Build history of the part. All positions in model axes, mm. Face numbers are marked on the shaded views. A direction names the side the tool comes from. Round coordinates to 2 decimals unless told otherwise and drop trailing zeros. Order: outer loops, then holes, each group sorted by start corner. A loop starts at its lowest first (then second) coordinate and runs counter-clockwise, first axis right, second up. Notation, with made-up numbers: (63, 81.25) -> (91, 81.25) arc R18 cw to (91, 98.25) -> close; hole circle Ø5 at (32.25, 85.5). An arc over 180 degrees is marked (long way). Answer as a JSON object with one key per item and string values.
from build123d import *

# Parameters (mm, degrees)
ESTRUSIONE_ESTRUSIONE1_DEPTH = 100
ESTRUSIONE_ESTRUSIONE2_DEPTH = 3


with BuildPart() as part:
    # Schizzo1 → Estrusione-Estrusione1 (new body)
    with BuildSketch(Plane(origin=(0, 0, 0), x_dir=(1, 0, 0), z_dir=(0, 1, 0))):
        Polygon((100, 0), (0, 0), (0, 220), (30, 220), (30, 225), (-5, 225), (-5, -5), (105, -5), (105, 30), (100, 30), align=None)
    extrude(amount=ESTRUSIONE_ESTRUSIONE1_DEPTH)

    # Schizzo2 → Estrusione-Estrusione2 (add)
    with BuildSketch(Plane.XZ):
        Polygon((30, -225), (-5, -225), (-5, 5), (105, 5), (105, -30), align=None)
    extrude(amount=-ESTRUSIONE_ESTRUSIONE2_DEPTH)


solid = part.part
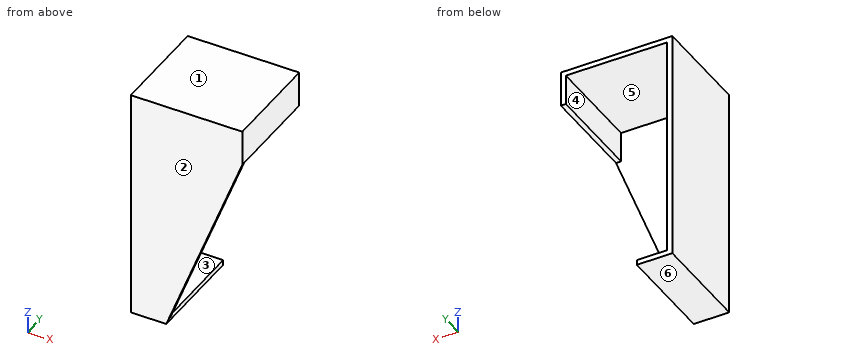
1) Pull direction Z, two halves, no side cores. Call the marked faces 1, 2 and 3: pulls with the +Z half, pulls with the -Z half, needs draft (parallel to the pull), parting line crosses it, or undercut.
Checked values:
{"face 1": "pulls with the +Z half", "face 2": "needs draft", "face 3": "undercut"}
2) Cut at A-A, the plane x = 15.5. Give the cut face in (y, z).
Checked values:
{"outline": "(0, -225) -> (100, -225) -> (100, -220) -> (3, -220) -> (3, 0) -> (100, 0) -> (100, 5) -> (0, 5) -> close"}
3) Flat gauge pins, fed straight in: pin 1 Ø10 at (y, z) = (42, -173) entering from +X; pin 2 Ø2.5 at (x, y) = (103, 66) entering from -Z; pin 3 Ø12 at (x, y) = (73, 63) entering from -Z. Where does each tip first touch, or does it go through?
Checked values:
{"pin 1": "stops at x = 0", "pin 2": "stops at z = -30", "pin 3": "stops at z = 0"}
4) Cut at C-C, the plane z = -15. Give the cut face in (x, y).
Checked values:
{"outline": "(-5, 0) -> (105, 0) -> (105, 100) -> (100, 100) -> (100, 3) -> (0, 3) -> (0, 100) -> (-5, 100) -> close"}
5) Cut at D-D, the plane x = 81.5. Give the cut face in (y, z).
Checked values:
{"outline": "(0, -91.1) -> (3, -91.1) -> (3, 0) -> (100, 0) -> (100, 5) -> (0, 5) -> close"}
6) Cut at B-B, the plane y = 14. Give the cut face in (x, z), plus the area to 4 significant figures.
Checked values:
{"outline": "(-5, -225) -> (30, -225) -> (30, -220) -> (0, -220) -> (0, 0) -> (100, 0) -> (100, -30) -> (105, -30) -> (105, 5) -> (-5, 5) -> close", "area": "1,975 mm²"}
7) Probe L1, parallel to X at y = 48.5, z = -9.5; L2, parallel to Z at x = 3, y = 62; L3, parallel to Z at x = 60, y = 73. List the from-to ranges inside material, lowest first. Write a range as from..to.
Checked values:
{"L1": "x = -5..0, 100..105", "L2": "z = -225..-220, 0..5", "L3": "z = 0..5"}
8) Which spindle directions (+Z, -Z, +X, -X, +Y, -Y) get a long thin tool onto all of the face, cutting with end or side? Do the marked faces 4, 5 and 6. Say none if no direction does.
Checked values:
{"face 4": "-Z, +Y", "face 5": "+Y", "face 6": "-Z, +X, -X, +Y, -Y"}
